Geometry check sheet. Reference: the model listing, model coordinates, mm. A direction names the side the tool comes from. Coordinates: 2 decimals unless noted, no trailing zeros. Order: outer loops, then holes, each group sorted by start corner. A loop starts at its lowest first (then second) coordinate and runs counter-clockwise, first axis right, second up. Notation, with made-up numbers: (55, 31.25) - (60, 31.25) arc R29 cw to (60, 65.25) - close; hole circle Ø6 at (-35, -12.75). An arc over 180 degrees is marked (long way). Return JSON: item names as keys, results as strings. Group by question number.
Item 1: Section check B-B on x = -2. Enter the section's corners in (y, z), then the cut area to 3 significant figures.
Item 2: Draft check along X on faces 3 (the flat face through (0, 0, 0)), 4 (the flat face through (0, -2, 0)), 5 (the cylindrical face through (-17, -1, 0)), 6 (the cylindrical face through (10.669, -1.485, 0.526)). Enter one of: pulls with the +X half, pulls with the -X half, needs draft (parallel to the pull), parting line crosses it, or undercut.
Item 3: Gauge pin test, flat ends, axial feed: pin 1 (1.5 mm diameter, centred on x = 10.5, y = -1, fed in from +Z); pin 2 (4 mm diameter, centred on x = 9, z = 0, fed in from -Y). Record the tip position at first contact, or that the pin passes through.
Item 4: Scan lines: probe 1 along X at (y, z) = (-2.15, -0.5); probe 2 along Z at (x, y) = (-9, -2.1); probe 3 along Z at (x, y) = (-9, -1.35). Record each from-to range of solid material in increasing order.
Item 5: Section check A-A on z = 0. Give the number of separate pieces and of enclosed holes in the cut face, then the cut area to 3 significant figures.
Item 6: Tool access check on faces 1 (the cylindrical face through (11.54, -2.49, -1.05)), 2 (the conical face through (-16.71, -1.89, 0.17)). Record the directions out of +Z, -Z, +X, -X, +Y, -Y that give a thin tool (end or side, any length) a straight path to the whole face; none if there is none.
from build123d import *

# Parameters (mm, degrees)
F0_R     = 1.75
F1_DEPTH = 2
F2_R     = 2.75
F2_R_2   = 1.75
F3_DEPTH = 1
F4_SIZE  = 0.4


with BuildPart() as f1:
    # F0 (on Front) → F1 (new body)
    with BuildSketch(Plane.XZ):
        with BuildLine():
            ThreePointArc((-9, 8), (-17, 0), (-9, -8))
            Line((-9, -8), (9, -8))
            ThreePointArc((9, -8), (17, 0), (9, 8))
            Line((9, 8), (-9, 8))
        make_face()
        with Locations((-9, 0)):
            Circle(F0_R, mode=Mode.SUBTRACT)
        with Locations((9, 0)):
            Circle(F0_R, mode=Mode.SUBTRACT)
    extrude(amount=F1_DEPTH)

    # F2 (on face) → F3 (join)
    with BuildSketch(Plane.XZ.offset(2)):
        with Locations((-9, 0)):
            Circle(F2_R)
        with Locations((-9, 0)):
            Circle(F2_R_2, mode=Mode.SUBTRACT)
        with Locations((9, 0)):
            Circle(F2_R)
        with Locations((9, 0)):
            Circle(F2_R_2, mode=Mode.SUBTRACT)
    extrude(amount=F3_DEPTH)

    # F4
    f4_edges = [f1.edges().sort_by_distance(p)[0] for p in [
        (-17, -2, 0),
        (0, -2, -8),
        (0, -2, 8),
        (17, -2, 0),
        (0, 0, 8),
        (-17, 0, 0),
        (0, 0, -8),
        (17, 0, 0),
        (-10.75, 0, 0),
        (7.25, 0, 0),
        (-10.75, -3, 0),
        (7.25, -3, 0),
    ]]
    chamfer(f4_edges, length=F4_SIZE)


solid = f1.part
Computed:
{
 "1": {"outline": "(-2, -7.6) - (-1.6, -8) - (-0.4, -8) - (0, -7.6) - (0, 7.6) - (-0.4, 8) - (-1.6, 8) - (-2, 7.6) - close", "area": "31.7 mm²"},
 "2": {"face 3": "needs draft", "face 4": "undercut", "face 5": "pulls with the -X half", "face 6": "undercut"},
 "3": {"pin 1": "stops at z = 7.96", "pin 2": "stops at y = -2.85"},
 "4": {"probe 1": "x = -11.7 to -10.68, -7.32 to -6.3, 6.3 to 7.32, 10.68 to 11.7", "probe 2": "z = -2.75 to -1.75, 1.75 to 2.75", "probe 3": "z = -8 to -1.75, 1.75 to 8"},
 "5": {"separate pieces": "3", "enclosed holes": "0", "area": "57.0 mm²"},
 "6": {"face 1": "-Y", "face 2": "-X, -Y"}
}
